Design review of the part built by this model. Coordinates are the model's own, in mm. Face numbers are marked on the shaded views. A direction names the side the tool comes from. Coordinates: 2 decimals unless noted, no trailing zeros. Write each loop counter-clockwise with the first axis right and the second up, starting at its lowest first coordinate (ties: lowest second). Pieces come first, ordered by that corner, then holes.
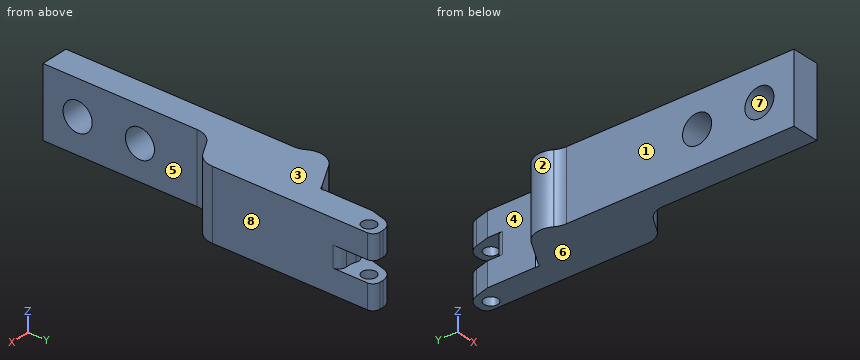
```python
from build123d import *

# Parameters (mm, degrees)
EXTRUDE_1_DEPTH     = 5
SKETCH_2_R          = 2.1
CUT_EXTRUDE_1_DEPTH = 53.575123334
SKETCH_3_R          = 1
SKETCH_3_R_2        = 0.5
CUT_EXTRUDE_2_DEPTH = 54.283614682
SKETCH_4_R          = 3
CUT_EXTRUDE_3_DEPTH = 1.5
FILLET_1_R          = 3
FILLET_4_R          = 1


with BuildPart() as part:
    # 草图1 → 凸台-拉伸1 (new, symmetric)
    with BuildSketch(Plane.XY):
        Polygon((-5.92820323, 37), (-4, 33.660254038), (-4, 0), (0, 0), (0, 24), (5, 26.886751346), (5, 52), (1, 52), (1, 41), align=None)
    extrude(amount=EXTRUDE_1_DEPTH, both=True)

    # 草图2 → 切除-拉伸1 (cut, through all)
    with BuildSketch(Plane(origin=(0, 0, 0), x_dir=(0, 0, -1), z_dir=(1, 0, 0))):
        with Locations((0, 14)):
            Circle(SKETCH_2_R)
        with Locations((0, 5)):
            Circle(SKETCH_2_R)
    extrude(amount=-CUT_EXTRUDE_1_DEPTH, mode=Mode.SUBTRACT)

    # 草图3 → 切除-拉伸2 (cut, through all)
    with BuildSketch(Plane.XY.offset(5)):
        with Locations((3.5, 50)):
            Circle(SKETCH_3_R)
        with Locations((0.566987298, 41.25)):
            Circle(SKETCH_3_R_2)
        with BuildLine():
            Line((3.5, 52), (5, 52))
            Line((5, 52), (5, 52.5))
            Line((5, 52.5), (1, 52.5))
            Line((1, 52.5), (1, 48.397279591))
            Line((1, 48.397279591), (1.568148347, 50.51763809))
            ThreePointArc((1.568148347, 50.51763809), (2.282477142, 51.586706681), (3.5, 52))
        make_face()
    extrude(amount=-CUT_EXTRUDE_2_DEPTH, mode=Mode.SUBTRACT)

    # 草图4 → 切除-拉伸3 (cut, symmetric)
    with BuildSketch(Plane.XY):
        with Locations((3.5, 50)):
            Circle(SKETCH_4_R)
    extrude(amount=CUT_EXTRUDE_3_DEPTH, both=True, mode=Mode.SUBTRACT)

    # 圆角1
    fillet_1_edges = [part.edges().sort_by_distance(p)[0] for p in [
        (0, 24, 0),
        (-4, 33.660254038, 0),
        (-5.92820323, 37, 0),
        (5, 26.886751346, 0),
    ]]
    fillet(fillet_1_edges, radius=FILLET_1_R)

    # 圆角4
    fillet_4_edges = [part.edges().sort_by_distance(p)[0] for p in [
        (5, 52, 3.25),
        (1, 48.341687605, 0),
        (5, 52, -3.25),
        (5, 47.401923789, 0),
    ]]
    fillet(fillet_4_edges, radius=FILLET_4_R)


solid = part.part
```
(1) Wall thickness on line 1 (Y direction, x = -2, z = 1); line 2 (Y direction, x = -1.3, z = 0); line 3 (Z direction, x = 2.5, y = 48): over which ranges is each line inside the solid? List them lowest first.
(2) Consider section D-D (y = 50). Give the boundary of the cut face in (x, z), plus the area to 3 significant figures.
(3) Consider section A-A (z = 3.25). Give the boundary of the cut face in (x, y).
(4) For the marked faces 1, 2, 3, 4 and 5, list the 3-axis set-ups (+Z, -Z, +X, -X, +Y, -Y) from which the entire face can be reached by the end or side of a thin tool; tool diameter is ignored.
(5) Consider section B-B (y = 14). Give the boundary of the cut face in (x, z), plus the area to 3 significant figures.
(6) Insertion check: pin 1 Ø5 at (y, z) = (39.5, -0.5) entering from -X; pin 2 Ø5 at (y, z) = (14, 0) entering from +X; pin 3 Ø3 at (y, z) = (28.5, 2.5) entering from -X; pin 4 Ø2.5 at (x, y) = (3.5, 50) entering from -Z. Each pin has a flat end and moves straight along its axis. Give the tip position at first contact, or say it passes through.
(7) Consider section C-C (z = 0). Give the boundary of the cut face in (x, y) (3 decimals).
(8) Mouldability with a two-part tool opening along Z and no side actions: class the marked faces 6, 7 and 8 as +Z half, -Z half, draft (parallel to the pull), parting line (faces both ways), or undercut.
Results:
1. line 1: y = 0 to 3.15, 6.85 to 12.15, 15.85 to 39.27
1. line 2: y = 0 to 2.9, 7.1 to 11.9, 16.1 to 39.67
1. line 3: z = -5 to -1.5, 1.5 to 5
2. outline: (1.43, -5) - (2.5, -5) - (2.5, -1.5) - (1.43, -1.5) - close; (1.43, 1.5) - (2.5, 1.5) - (2.5, 5) - (1.43, 5) - close; (4.5, -5) - (5, -5) - (5, -1.5) - (4.5, -1.5) - close; (4.5, 1.5) - (5, 1.5) - (5, 5) - (4.5, 5) - close
2. area: 11.0 mm2
3. outline: (-4.43, 34.4) - (-4.4, 34.36) arc R3 cw to (-4, 32.86) - (-4, 0) - (0, 0) - (0, 22.27) arc R3 cw to (1.5, 24.87) - (3.5, 26.02) arc R3 ccw to (5, 28.62) - (5, 51) arc R1 ccw to (4, 52) - (3.5, 52) arc R2 ccw to (1.57, 50.52) - (1, 48.4) - (1, 41.5) arc R0.5 cw to (0.57, 40.75) - (-3.33, 38.5) arc R3 ccw to start; hole circle Ø2 at (3.5, 50)
4. face 1: +Z, -Z, -X, -Y
4. face 2: +Z, -Z, -X
4. face 3: +Z, +X, -X, +Y, -Y
4. face 4: +Z, -Z, -X, +Y
4. face 5: +Z, -Z, +X, -Y
5. outline: (-4, -5) - (0, -5) - (0, -2.1) - (-4, -2.1) - close; (-4, 2.1) - (0, 2.1) - (0, 5) - (-4, 5) - close
5. area: 23.2 mm2
6. pin 1: stops at x = -4.62
6. pin 2: stops at x = 0
6. pin 3: stops at x = -4
6. pin 4: stops at z = -5
7. outline: (-4.428, 34.402) - (-4.402, 34.356) arc R3 cw to (-4, 32.856) - (-4, 16.1) - (0, 16.1) - (0, 22.268) arc R3 cw to (1.5, 24.866) - (3.5, 26.021) arc R3 ccw to (5, 28.619) - (5, 46.031) arc R1 ccw to (3.875, 47.024) arc R3 cw to (2.375, 47.219) arc R1 ccw to (1, 46.292) - (1, 41.5) arc R0.5 cw to (0.567, 40.75) - (-3.33, 38.5) arc R3 ccw to start; (-4, 0) - (0, 0) - (0, 2.9) - (-4, 2.9) - close; (-4, 7.1) - (0, 7.1) - (0, 11.9) - (-4, 11.9) - close
8. face 6: -Z half
8. face 7: undercut
8. face 8: draft
